Read the model definition and answer for the solid it produces. Units are mm, in the model's axes. Coordinates: 2 decimals unless noted, no trailing zeros. Loops run counter-clockwise (first coordinate to the right, second up) from the corner with the lowest first, then second, coordinate; pieces in that order, holes last. Notation, with made-up numbers: (85, -21) - (134, -21) arc R17 ccw to (134, -5) - close; hole circle Ø3 at (42.25, 2). An arc over 180 degrees is marked (long way). Use CSV: the item, a comma, the result in double quotes.
```python
from build123d import *

# Parameters (mm, degrees)
F0_R     = 25.627184
F1_DEPTH = 164
F2_R     = 3.189044
F2_R_2   = 3.059411
F2_R_3   = 4.263801
F2_R_4   = 3.084232
F3_DEPTH = 137
F4_R     = 4.101554
F4_R_2   = 6.872634
F4_R_3   = 5.28999
F4_R_4   = 5.785283
F5_DEPTH = 152


with BuildPart() as f1:
    # F0 (on Top) → F1 (new body)
    with BuildSketch(Plane.XY):
        Circle(F0_R)
    extrude(amount=F1_DEPTH)

    # F2 (on face) → F3 (join)
    with BuildSketch(Plane(origin=(0, 0, 0), x_dir=(1, 0, 0), z_dir=(0, 0, -1))):
        with Locations((-8.850001, 14.700001)):
            Circle(F2_R)
        with Locations((7.950001, 13.200001)):
            Circle(F2_R_2)
        with Locations((9.750001, -4.8)):
            Circle(F2_R_3)
        with Locations((-4.950002, -7.5)):
            Circle(F2_R_4)
    extrude(amount=F3_DEPTH)

    # F4 (on face) → F5 (join)
    with BuildSketch(Plane.XY.offset(164)):
        with Locations((-9.454723, 15.175114)):
            Circle(F4_R)
        with Locations((6.632895, 9.544446)):
            Circle(F4_R_2)
        with Locations((5.828514, -11.771653)):
            Circle(F4_R_3)
        with Locations((-15.085398, 0)):
            Circle(F4_R_4)
    extrude(amount=F5_DEPTH)


solid = f1.part
```
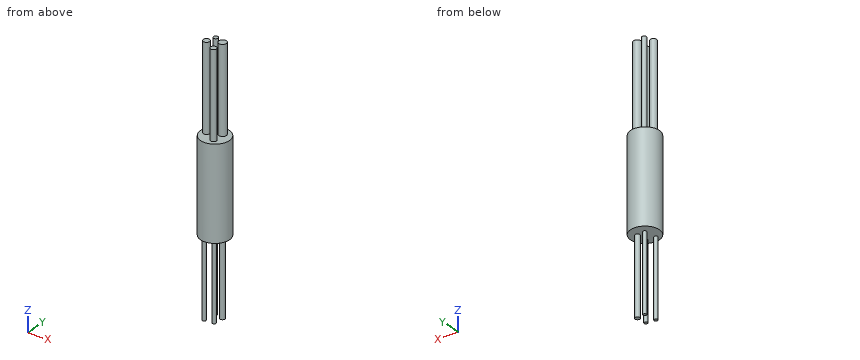
Q1. The part is cut by section A-A on z = -44.5. Determine the outline of the cut face in (x, y), and give its area (3 significant figures).
Reported:
outline,"circle Ø6.38 at (-8.85, -14.7); circle Ø6.17 at (-4.95, 7.5); circle Ø6.12 at (7.95, -13.2); circle Ø8.53 at (9.75, 4.8)"
area,"148 mm²"
Q2. Given P1, Ø8, axis at x = 1, y = 16, coming from the -Z side; P2, Ø8, axis at x = -13, z = 141.5, coming from the -Y side; P3, Ø5, axis at y = 4, z = 197, coming from the +X side, each flat-ended and moving along its own axis, determine where each tip first touches the part or whether it passes through.
Reported:
P1,"stops at z = 0"
P2,"stops at y = -23.99"
P3,"stops at x = 12.79"
Q3. The part is cut by section C-C on z = 174. Determine the outline of the cut face in (x, y).
Reported:
outline,"circle Ø11.57 at (-15.09, 0); circle Ø8.2 at (-9.45, 15.18); circle Ø13.75 at (6.63, 9.54); circle Ø10.58 at (5.83, -11.77)"
Q4. Find the intervals of material crossed by probe 1 along Z at (x, y) = (-8, 16.5); probe 2 along Z at (x, y) = (3.5, -2); probe 3 along X at (y, z) = (-0.5, 90), in increasing order. Write a range as [from, to].
Reported:
probe 1,"z = [0, 316]"
probe 2,"z = [0, 164]"
probe 3,"x = [-25.62, 25.62]"
Q5. The part is cut by section B-B on z = 118. Determine the outline of the cut face in (x, y).
Reported:
outline,"circle Ø51.25 at (0, 0)"
